```python
from build123d import *

# Parameters (mm, degrees)
F1_DEPTH = 3
F2_R     = 2.5
F3_DEPTH = 25
F5_DEPTH = 1
F6_SIZE  = 0.99999


# Not quite as in the source:
# - a fillet or chamfer is up to 0.001 mm smaller than in the source, because OpenCascade refuses the exact size


with BuildPart() as f1:
    # F0 (on Top) → F1 (new body)
    with BuildSketch(Plane.XY):
        with BuildLine():
            Line((-7.0720659795, 18.1059757224), (-16.646664491, 0))
            ThreePointArc((-16.646664491, 0), (0, -27.6337946959), (16.646664491, 0))
            Line((16.646664491, 0), (7.0720659795, 18.1059757224))
            ThreePointArc((7.0720659795, 18.1059757224), (0, 22.3662053041), (-7.0720659795, 18.1059757224))
        make_face()
    extrude(amount=F1_DEPTH)

    # F2 (on face) → F3 (cut)
    with BuildSketch(Plane.XY.offset(3)):
        with Locations((0, 14.3662053041)):
            Circle(F2_R)
    extrude(amount=-F3_DEPTH, mode=Mode.SUBTRACT)

    # F4 (on face) → F5 (cut)
    with BuildSketch(Plane.XY.offset(3)):
        with BuildLine():
            Line((15.7626562435, -0.4674713023), (6.1880577321, 17.6385044201))
            ThreePointArc((6.1880577321, 17.6385044201), (0, 21.3662053041), (-6.1880577321, 17.6385044201))
            Line((-6.1880577321, 17.6385044201), (-15.7626562435, -0.4674713023))
            ThreePointArc((-15.7626562435, -0.4674713023), (0, -26.6337946959), (15.7626562435, -0.4674713023))
        make_face()
    extrude(amount=-F5_DEPTH, mode=Mode.SUBTRACT)

    # F6 (size 1 in the source; OpenCascade refuses exactly that, so slightly less here)
    f6_edges = [f1.edges().sort_by_distance(p)[0] for p in [
        (0, -26.633795, 2),
        (-10.975357, 8.585517, 2),
        (10.975357, 8.585517, 2),
        (0, 21.366205, 2),
        (-2.5, 14.366205, 2),
    ]]
    chamfer(f6_edges, length=F6_SIZE)


solid = f1.part
```
Read the model definition and answer for the solid it produces. Units are mm, in the model's axes. A direction names the side the tool comes from. Give positions to 0.01 mm unless a question says otherwise; leave off trailing zeros. Write item = value, one per line.
1. Straight lines are drawn through the part: line 1 along Y through (x, z) = (4, 2.95); line 2 along Z through (x, y) = (0, -22.5); line 3 along X through (y, z) = (5.5, 2.15). For each, find the intervals that lie inside material, in ascending order.
Numbers:
line_1 = -27.2 to -26.13, 20.05 to 21.29
line_2 = 0 to 2
line_3 = -13.74 to -11.65, 11.65 to 13.74
2. The mould has two halves that part along X. Classify faces 1 (the face through (15.3, 1.2, 3)), 2 (the face through (-0.542, -27.626, 1.479)), 3 (the face through (-10.46, 8.475, 2.493)): +X half, -X half, draft (parallel to the pull), parting line (faces both ways), or undercut.
Numbers:
face_1 = draft
face_2 = parting line
face_3 = undercut
3. Given pin 1 (10 mm diameter, centred on x = 0, y = -5.5, fed in from +Z); pin 2 (8 mm diameter, centred on x = 4.5, y = 17, fed in from -Z), each flat-ended and moving along its own axis, determine where each tip first touches the part or whether it passes through.
Numbers:
pin_1 = 2
pin_2 = 0
4. For faces 4 (the face through (0.094, 20.525, 2.16)), 5 (the face through (0, -2, 0)), determine the directions among +Z, -Z, +X, -X, +Y, -Y from which every point of the face is accessible in a straight line to the end or side of a thin tool.
Numbers:
face_4 = +Z
face_5 = -Z, +X, -X, +Y, -Y
